Autodesk Fusion 360 part; units mm, degrees
sketch "Main cross-section sketch" plane through (0, 0, 0) normal (0, 1, 0) x (1, 0, 0)
  line L0 (6.1, -6.1) -> (-6.1, -6.1)
  line L1 (-6.1, -6.1) -> (-6.1, 6.1)
  line L2 (-6.1, 6.1) -> (6.1, 6.1)
  line L3 (6.1, 6.1) -> (6.1, -6.1)
  line L4 (29.75, -10.1) -> (-29.75, -10.1)
  line L5 (-29.75, -10.1) -> (-31.5173, 10.1)
  line L6 (-31.5173, 10.1) -> (31.5173, 10.1)
  line L7 (31.5173, 10.1) -> (29.75, -10.1)
  line L8 (-29.75, -10.1) -> (29.75, -10.1)
  line L9 (-6.1, -6.1) -> (-30.1, -6.1) construction
  line L10 (6.1, -6.1) -> (30.1, -6.1) construction
  line L11 (6.1, -6.1) -> (-6.1, 6.1) construction
  line L12 (6.1, 6.1) -> (-6.1, -6.1) construction
  dimension "d13" = 85
  dimension "d14" = 85
  dimension "d20" = 24
  dimension "d22" = 4
  dimension "d25" = 4
  dimension "d26" = 12.2
extrude "Extrude1" add sketch "Main cross-section sketch" along normal blind 100 makes body 1
sketch "Right side sketch" plane through (30.401, 0, 2.6597) normal (0.9962, 0, 0.0872) x (0, 1, 0)
  line L0 (0, 7.4687) -> (0, -12.8085)
  line L1 (0, -12.8085) -> (100, -12.8085)
  line L2 (100, -12.8085) -> (100, 7.4687)
  line L3 (100, 7.4687) -> (0, 7.4687)
  circle A0 centre (9, -2.6699) radius 4.825
  circle A1 centre (92.0226, -4.7633) radius 3.24
  line L4 (9, -2.6699) -> (0, -2.6699) construction
  line L5 (9, -2.6699) -> (92.0226, -2.6699) construction
  line L6 (92.0226, -2.6699) -> (100, -2.6699) construction
  dimension "d31" = 9.65
  dimension "d32" = 6.48
  dimension "d44" = 9
  dimension "d64" = 2.0934
  dimension "d65" = 83.0226
extrude "Extrude5" add sketch "Right side sketch" along normal blind 20 contours A0 | A1 bodies 1
mirror "Mirror1" about plane through (0, 0, 0) normal (1, 0, 0) of "Extrude5"
extrude "Extrude6" add sketch "Right side sketch" along normal blind 20 bodies 1
extrude "Extrude7" add 1 faces at (-30.2168, 67.337, 4.7654) along direction (-0.996195, 0, 0.087156) blind 20 on bodies 1 bodies 1
split "Split1" by plane through (0, 0, 0) normal (0, 0, 1) bodies 1 makes body 2 at (-10.5058, 33.3333, -10.1)
move_body "Move1" bodies 2 to x (-1, 0, 0) y (0, 1, 0) z (0, 0, -1) at (62.2, 0, 0.2)
delete_body "RemoveBody1" bodies 1
delete_body "RemoveBody2" bodies 2
extrude "Extrude8" add sketch "Main cross-section sketch" along normal blind 100 separate body makes body 3
extrude "Extrude9" cut sketch "Right side sketch" against normal blind 20 contours A0 | A1 bodies 3
mirror "Mirror2" about plane through (0, 0, 0) normal (1, 0, 0) of "Extrude9"
extrude "Extrude4" [suppressed]
extrude "Extrude2" [suppressed]
sketch "Left side sketch" plane through (-11.8041, 0, 1.0327) normal (-0.9962, 0, 0.0872) x (0, -1, 0)
  line L0 (0, -9.9817) -> (0, 8.2879)
  line L1 (0, 8.2879) -> (-100, 8.2879)
  line L2 (-100, 8.2879) -> (-100, -9.9817)
  line L3 (-100, -9.9817) -> (0, -9.9817)
  circle A0 centre (-92.0226, -2.9403) radius 5.19
  circle A1 centre (-92.0226, -2.9403) radius 3.19
  circle A2 centre (-9, -0.8469) radius 4.775
  circle A3 centre (-9, -0.8469) radius 6.775
  line L4 (-100, -0.8469) -> (0, -0.8469) construction
  dimension "d40" = 9.55
  dimension "d41" = 6.38
  dimension "d42" = 13.55
  dimension "d43" = 10.38
  dimension "d47" = 9
  dimension "d66" = 2.0934
  dimension "d67" = 83.0226
extrude "Extrude3" [suppressed]
hole "Hole1" [suppressed]
hole "Hole2" [suppressed]
hole "Hole3" [suppressed]
hole "Hole4" [suppressed]
equation "d42 = 9.55 mm + 4 mm"
equation "d43 = 6.38 mm + 4 mm"
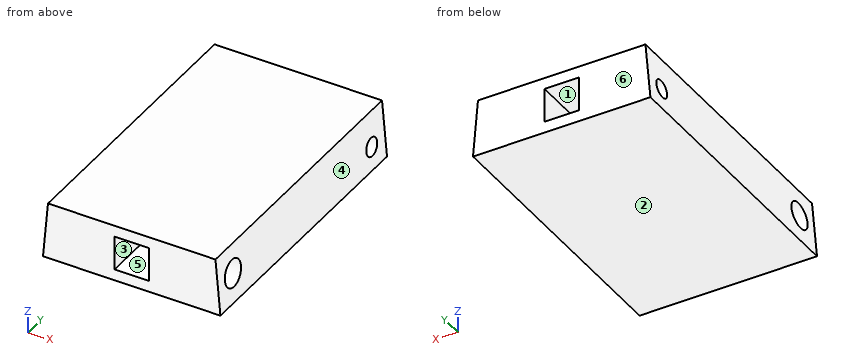
Work out the finished part from the listing and answer in its coordinate system (mm). Face numbers are marked on the shaded views. A direction names the side the tool comes from. Round coordinates to 2 decimals unless told otherwise and drop trailing zeros. Loops run counter-clockwise (first coordinate to the right, second up) from the corner with the lowest first, then second, coordinate; pieces in that order, holes last. Notation, with made-up numbers: (29, 63.25) - (58, 63.25) arc R34 ccw to (58, 94.25) - close; hole circle Ø7 at (-7, 10.25). An arc over 180 degrees is marked (long way). Use one line per item in the form item = value. Start each with the question number.
(1) Consider line 1 (Z direction, x = 4, y = 83.5); line 2 (Y direction, x = 14, z = -3.5); line 3 (Y direction, x = -12, z = -2.5). Determine where each line is inside the solid, lowest interval first.
(2) Determine the mould class of the marked faces 3, 4, 5 and 6 for opening direction Z: +Z half, -Z half, draft (parallel to the pull), parting line (faces both ways), or undercut.
(3) Find section C-C on y = 90. Determine the outline of the cut face in (x, z).
(4) Find section A-A on x = -5. Determine the outline of the cut face in (y, z).
(5) Which of the six approach directions +Z, -Z, +X, -X, +Y, -Y give full straight-line access (tool end or side, diameter ignored) to the marked faces 1 and 2?
(6) Flat-ended cylindrical pins translate along their axes: P1, Ø4, axis at y = 19, z = -4.5, coming from the +X side; P2, Ø1.5, axis at y = 47.5, z = -6.5, coming from the +X side; P3, Ø8, axis at y = 50.5, z = -0.5, coming from the +X side. Find the tip coordinate at first contact, or state that the pin passes through.
(7) Find section B-B on y = 39. Determine the outline of the cut face in (x, z), and give its area (3 significant figures).
(8) Find section D-D on x = 14.5. Give the number of separate pieces and of enclosed holes in the cut face, and give its area (3 significant figures).
Answer list:
q1.line_1 = -10.1 to -6.1, 6.1 to 10.1
q1.line_2 = 0 to 4.63, 13.37 to 88.78, 95.26 to 100
q1.line_3 = 0 to 4.25, 13.75 to 89.02, 95.02 to 100
q2.face_3 = undercut
q2.face_4 = +Z half
q2.face_5 = undercut
q2.face_6 = draft
q3.outline = (-31.52, -10.1) - (31.52, -10.1) - (31.04, -4.61) - (11.11, -6.35) - (10.67, -1.31) - (30.6, 0.44) - (29.75, 10.1) - (-29.75, 10.1) - (-30.6, 0.44) - (-10.67, -1.31) - (-11.11, -6.35) - (-31.04, -4.61) - close; hole (-6.1, -6.1) - (6.1, -6.1) - (6.1, 6.1) - (-6.1, 6.1) - close
q4.outline = (0, -10.1) - (100, -10.1) - (100, -6.1) - (0, -6.1) - close; (0, 6.1) - (100, 6.1) - (100, 10.1) - (0, 10.1) - close
q5.face_1 = +Y, -Y
q5.face_2 = -Z, +X, -X, +Y, -Y
q6.P1 = 31.2
q6.P2 = 31.27
q6.P3 = 31.03
q7.outline = (-31.52, -10.1) - (31.52, -10.1) - (29.75, 10.1) - (-29.75, 10.1) - close; hole (-6.1, -6.1) - (6.1, -6.1) - (6.1, 6.1) - (-6.1, 6.1) - close
q7.area = 1,090 mm^2
q8.separate_pieces = 1
q8.enclosed_holes = 2
q8.area = 1,910 mm^2
